The listing builds one solid part. Answer for the finished solid, in the listing's coordinates (mm). A direction names the side the tool comes from. Coordinates: 2 decimals unless noted, no trailing zeros. Order: outer loops, then holes, each group sorted by start corner. A loop starts at its lowest first (then second) coordinate and runs counter-clockwise, first axis right, second up. Notation, with made-up numbers: (21, 66) - (62, 66) arc R21 cw to (62, 86) - close; hole circle Ø11 at (87, 35.5). An arc over 180 degrees is marked (long way). Use a Markdown table: item, result. Add a question column.
Item 1: The mould has two halves that part along Y. Classify faces 1 (the cylindrical face through (3.8, -18.553, 3.451)), 2 (the cylindrical face through (-11.79, 12.13, 3.45)), 3 (the flat face through (-9, -10, 7)): released by +Y, released by -Y, zero draft, split by the parting line, or undercut.
Item 2: Find the intervals of material crossed by line 1 along Y through (x, z) = (9, 1.25); line 2 along X through (y, z) = (-9, 6.5); line 3 along X through (y, z) = (-3, 0.5), in increasing order.
Item 3: Flat-ended cylindrical pins translate along their axes: P1, Ø16, axis at x = 0, y = 0, coming from the +Z side; P2, Ø1.5, axis at y = 31, z = 3, coming from the +X side; P3, Ø1, axis at y = 10.5, z = 5, coming from the -X side. Find the tip coordinate at first contact, or state that the pin passes through.
Item 4: The part is cut by section C-C, the plane x = -6. Give the vertices of the cut face in (y, z).
Item 5: For faces 4 (the cylindrical face through (-1.458, 37.866, 3.451)), 5 (the cylindrical face through (11.87, 10.58, 3.45)), determine the directions among +Z, -Z, +X, -X, +Y, -Y from which every point of the face is accessible in a straight line to the end or side of a thin tool.
Item 6: The part is cut by section A-A, the plane x = -23.5. Give the vertices of the cut face in (y, z).
Item 7: The part is cut by section B-B, the plane y = -3. Give the vertices of the cut face in (x, z), then the cut area to 3 significant figures.
Item 8: The part is cut by section D-D, the plane z = 5.25. Give the vertices of the cut face in (x, y), then the cut area to 3 significant figures.
from build123d import *

# Parameters (mm, degrees)
F0_R     = 11.2
F1_DEPTH = 7


with BuildPart() as f1:
    # F0 (on Top) → F1 (new body)
    with BuildSketch(Plane.XY):
        with BuildLine():
            ThreePointArc((10.140133, -8.450899), (-12.411482, 4.493898), (13.2, 0))
            ThreePointArc((13.2, 0), (12.977457, -2.413629), (12.317332, -4.745875))
            ThreePointArc((12.317332, -4.745875), (16.727086, -1.305485), (22.165645, 0))
            ThreePointArc((22.165645, 0), (18.992247, 3.053889), (18.446518, 7.424114))
            ThreePointArc((18.446518, 7.424114), (11.802919, 10.656167), (9.608782, 17.710905))
            ThreePointArc((9.608782, 17.710905), (-0.841952, 13.588271), (-10.682802, 19.007829))
            ThreePointArc((-10.682802, 19.007829), (-11.862909, 12.054078), (-18.776167, 10.656167))
            ThreePointArc((-18.776167, 10.656167), (-16.394376, 5.178266), (-18.282297, -0.488839))
            ThreePointArc((-18.282297, -0.488839), (-12.387933, -5.351975), (-10.176054, -12.666426))
            ThreePointArc((-10.176054, -12.666426), (-10.605131, -16.004618), (-11.864467, -19.125788))
            ThreePointArc((-11.864467, -19.125788), (-4.683804, -17.813616), (0, -23.412337))
            ThreePointArc((0, -23.412337), (3.878012, -18.508514), (10.09119, -17.813616))
            ThreePointArc((10.09119, -17.813616), (9.257646, -13.127772), (10.140133, -8.450899))
        make_face()
        with BuildLine():
            ThreePointArc((12.317332, -4.745875), (11.38052, -6.687582), (10.140133, -8.450899))
            ThreePointArc((10.140133, -8.450899), (9.257646, -13.127772), (10.09119, -17.813616))
            ThreePointArc((10.09119, -17.813616), (24.803224, -26.186671), (35.657465, -13.196774))
            ThreePointArc((35.657465, -13.196774), (31.687524, -3.760354), (22.165645, 0))
            ThreePointArc((22.165645, 0), (16.727086, -1.305485), (12.317332, -4.745875))
        make_face()
        with Locations((22.457465, -13.196774)):
            Circle(F0_R, mode=Mode.SUBTRACT)
        with BuildLine():
            ThreePointArc((-18.282297, -0.488839), (-35.856773, -16.964294), (-11.864467, -19.125788))
            ThreePointArc((-11.864467, -19.125788), (-10.605131, -16.004618), (-10.176054, -12.666426))
            ThreePointArc((-10.176054, -12.666426), (-12.387933, -5.351975), (-18.282297, -0.488839))
        make_face()
        with Locations((-23.376054, -12.666426)):
            Circle(F0_R, mode=Mode.SUBTRACT)
        with BuildLine():
            ThreePointArc((-10.682802, 19.007829), (-0.841952, 13.588271), (9.608782, 17.710905))
            ThreePointArc((9.608782, 17.710905), (12.269391, 21.892918), (13.2, 26.761392))
            ThreePointArc((13.2, 26.761392), (-3.287299, 39.54551), (-11.562677, 20.393935))
            ThreePointArc((-11.562677, 20.393935), (-11.076889, 19.729987), (-10.682802, 19.007829))
        make_face()
        with Locations((0, 26.761392)):
            Circle(F0_R, mode=Mode.SUBTRACT)
        with BuildLine():
            ThreePointArc((-11.562677, 20.393935), (-11.14431, 19.687189), (-10.682802, 19.007829))
            ThreePointArc((-10.682802, 19.007829), (-11.076889, 19.729987), (-11.562677, 20.393935))
        make_face()
    extrude(amount=F1_DEPTH)


solid = f1.part
Solution:
| question | item | result |
|---|---|---|
| 1 | face 1 | released by -Y |
| 1 | face 2 | undercut |
| 1 | face 3 | zero draft |
| 2 | line 1 | y = -17.58 to -9.66, 9.66 to 20.1, 33.43 to 36.42 |
| 2 | line 2 | x = -36.06 to -33.96, -12.79 to -9.66, 9.66 to 12.07, 32.84 to 34.97 |
| 2 | line 3 | x = -32.36 to -29.03, -17.72 to -12.85, 12.85 to 17.82, 27.09 to 30.84 |
| 3 | P1 | passes through |
| 3 | P2 | stops at x = 12.73 |
| 3 | P3 | stops at x = -18.78 |
| 4 | outline | (-17.47, 0) - (-11.76, 0) - (-11.76, 7) - (-17.47, 7) - close; (11.76, 0) - (17.3, 0) - (17.3, 7) - (11.76, 7) - close; (36.22, 0) - (38.52, 0) - (38.52, 7) - (36.22, 7) - close |
| 5 | face 4 | +Z, -Z |
| 5 | face 5 | +Z, -Z, +X |
| 6 | outline | (-25.87, 0) - (-23.87, 0) - (-23.87, 7) - (-25.87, 7) - close; (-1.47, 0) - (0.53, 0) - (0.53, 7) - (-1.47, 7) - close |
| 7 | outline | (-32.36, 0) - (-29.03, 0) - (-29.03, 7) - (-32.36, 7) - close; (-17.72, 0) - (-12.85, 0) - (-12.85, 7) - (-17.72, 7) - close; (12.85, 0) - (17.82, 0) - (17.82, 7) - (12.85, 7) - close; (27.09, 0) - (30.84, 0) - (30.84, 7) - (27.09, 7) - close |
| 7 | area | 118 mm2 |
| 8 | outline | (-18.78, 10.66) arc R8.35 cw to (-18.28, -0.49) arc R13.2 ccw (long way) to (-11.86, -19.13) arc R7.25 cw to (0, -23.41) arc R8.12 cw to (10.09, -17.81) arc R13.2 ccw to (35.66, -13.2) arc R13.2 ccw to (22.17, 0) arc R6.6 cw to (18.45, 7.42) arc R9.3 cw to (9.61, 17.71) arc R13.2 ccw to (13.2, 26.76) arc R13.2 ccw (long way) to (-11.56, 20.39) arc R13.2 ccw to (-10.68, 19.01) arc R6.23 cw to start; hole circle Ø22.4 at (-23.38, -12.67); hole circle Ø22.4 at (0, 26.76); hole (10.14, -8.45) arc R13.2 ccw to (12.32, -4.75) arc R13.2 ccw to (13.2, 0) arc R13.2 ccw (long way) to start; hole circle Ø22.4 at (22.46, -13.2) |
| 8 | area | 809 mm2 |
